Autodesk Inventor part; units mm, degrees
ref_plane "c1_XY" through (22.225, 7.9057, 0) normal (0, 0, 1) x (1, 0, 0)
ref_plane "c1_YZ" through (22.225, 7.9057, 0) normal (1, 0, 0) x (0, 1, 0)
ref_plane "c1_ZX" through (22.225, 7.9057, 0) normal (0, 1, 0) x (0, 0, 1)
sketch "Sketch_18" plane through (0, 0, 0) normal (0, 0, 1) x (1, 0, 0)
  line L0 (22.225, 0) -> (0, 0)
  line L1 (0, 0) -> (0, 12.846)
  line L2 (0, 12.846) -> (0.762, 13.6081)
  line L3 (0.762, 13.6081) -> (4.826, 13.6081)
  line L4 (4.826, 13.6081) -> (5.588, 12.846)
  line L5 (5.588, 12.846) -> (6.35, 12.846)
  line L6 (6.35, 12.846) -> (6.35, 14.1097)
  line L7 (6.35, 14.1097) -> (21.463, 14.1097)
  line L8 (21.463, 14.1097) -> (22.225, 13.3477)
  line L9 (22.225, 13.3477) -> (22.225, 0)
  line L10 (22.225, 0) -> (0, 0)
revolve "Revolution1" add sketch "Sketch_18" angle 360 about axis through (22.225, 0, 0) along (1, 0, 0)
sketch "Sketch_15" plane through (0, 0, 0) normal (0, 0, 1) x (1, 0, 0)
  line L0 (38.1, 0) -> (22.225, 0)
  line L1 (22.225, 0) -> (22.225, 7.9057)
  line L2 (22.225, 7.9057) -> (24.6126, 7.9057)
  line L3 (24.6126, 7.9057) -> (24.6126, 7.7279)
  arc A0 (24.6126, 7.7279) -> (25.5016, 6.839) centre (25.5016, 7.7279) ccw
  line L4 (25.5016, 6.839) -> (26.7843, 6.839)
  arc A1 (26.7843, 6.839) -> (27.383, 7.0708) centre (26.7843, 7.7279) ccw
  line L5 (27.383, 7.0708) -> (27.4129, 7.098)
  line L6 (27.4129, 7.098) -> (28.2524, 7.9375)
  line L7 (28.2524, 7.9375) -> (37.2605, 7.9375)
  line L8 (37.2605, 7.9375) -> (38.1, 7.098)
  line L9 (38.1, 7.098) -> (38.1, 0)
  line L10 (38.1, 0) -> (22.225, 0)
revolve "Revolution2" add sketch "Sketch_15" angle 360 about axis through (38.1, 0, 0) along (1, 0, 0)
thread "Thread1"
sketch "Sketch_9" plane through (38.1, 0, 0) normal (1, 0, 0) x (0, 0, -1)
  line L0 (-28.2194, -56.4388) -> (28.2194, -56.4388)
  line L1 (28.2194, -56.4388) -> (28.2194, 56.4388)
  line L2 (28.2194, 56.4388) -> (-28.2194, 56.4388)
  line L3 (-28.2194, 56.4388) -> (-28.2194, -56.4388)
  line L4 (-4.7307, -28.2194) -> (4.7307, -28.2194)
  line L5 (4.7307, -28.2194) -> (4.7307, 28.2194)
  line L6 (4.7307, 28.2194) -> (-4.7307, 28.2194)
  line L7 (-4.7307, 28.2194) -> (-4.7307, -28.2194)
extrude "Extrusion1" cut sketch "Sketch_9" against normal blind 15.875
sketch "Sketch_13" plane through (0, 0, 0) normal (0, 0, 1) x (1, 0, 0)
  line L0 (21.7996, 0) -> (0, 0)
  line L1 (0, 0) -> (0, 4.7625)
  line L2 (0, 4.7625) -> (19.05, 4.7625)
  line L3 (19.05, 4.7625) -> (21.7996, 0)
  line L4 (21.7996, 0) -> (0, 0)
revolve "Revolution3" cut sketch "Sketch_13" angle 360 about axis through (21.7996, 0, 0) along (1, 0, 0)
sketch "Sketch_19" plane through (0, 0, 0) normal (0, 1, 0) x (-1, 0, 0)
  line L0 (-15.0876, 14.1097) -> (-15.0876, 0)
  line L1 (-15.0876, 0) -> (-19.6754, 0)
  line L2 (-19.6754, 0) -> (-19.6754, 6.0491)
  line L3 (-19.6754, 6.0491) -> (-19.9073, 13.4747)
  line L4 (-19.9073, 13.4747) -> (-20.5423, 14.1097)
  line L5 (-20.5423, 14.1097) -> (-15.0876, 14.1097)
  line L6 (-15.0876, 14.1097) -> (-15.0876, 0)
revolve "Revolution4" cut sketch "Sketch_19" angle 360 about axis through (15.0876, 0, 14.1097) along (0, 0, 1)
sketch "Sketch_24" plane through (0, 0, 0) normal (0, 0, 1) x (1, 0, 0)
  line L0 (6.35, 0) -> (5.588, 0)
  line L1 (5.4861, 14.0255) -> (6.2275, 13.2842)
  arc A0 (6.2275, 13.1046) -> (6.2275, 13.2842) centre (6.1377, 13.1944) ccw
  line L2 (6.2275, 13.1046) -> (5.969, 12.846)
  line L3 (5.969, 12.846) -> (5.588, 12.846)
  line L4 (5.588, 12.846) -> (5.588, 12.5921)
  line L5 (5.588, 12.5921) -> (6.35, 12.5921)
  line L6 (6.35, 12.5921) -> (6.35, 13.449)
  line L7 (6.35, 13.449) -> (5.6893, 14.1097)
  line L8 (5.6893, 14.1097) -> (5.4861, 14.1097)
  line L9 (5.4861, 14.1097) -> (5.4861, 14.0255)
revolve "Revolution5" add sketch "Sketch_24" angle 360 about axis through (6.35, 0, 0) along (1, 0, 0)
sketch "Sketch_43" plane through (0, 0, 0) normal (0, 0, 1) x (1, 0, 0)
  circle A0 centre (30.9626, 0) radius 3.2004
extrude "Extrusion2" cut sketch "Sketch_43" along normal mid plane 14.1922
ref_plane "c1_XY" through (22.225, 7.9057, 0) normal (0, 0, 1) x (1, 0, 0)
ref_plane "c1_YZ" through (22.225, 7.9057, 0) normal (1, 0, 0) x (0, 1, 0)
ref_plane "c1_ZX" through (22.225, 7.9057, 0) normal (0, 1, 0) x (0, 0, 1)
ref_plane "cc1_XY" through (22.225, 0, 0) normal (0, 0, 1) x (1, 0, 0)
ref_plane "cc1_YZ" through (22.225, 0, 0) normal (1, 0, 0) x (0, 1, 0)
ref_plane "cc1_ZX" through (22.225, 0, 0) normal (0, 1, 0) x (0, 0, 1)
ref_plane "c2_XY" through (22.225, -7.9057, 0) normal (0, 0, 1) x (1, 0, 0)
ref_plane "c2_YZ" through (22.225, -7.9057, 0) normal (1, 0, 0) x (0, 1, 0)
ref_plane "c2_ZX" through (22.225, -7.9057, 0) normal (0, 1, 0) x (0, 0, 1)
ref_plane "cc2_XY" through (24.6126, 0, 0) normal (0, 0, 1) x (1, 0, 0)
ref_plane "cc2_YZ" through (24.6126, 0, 0) normal (1, 0, 0) x (0, 1, 0)
ref_plane "cc2_ZX" through (24.6126, 0, 0) normal (0, 1, 0) x (0, 0, 1)
ref_plane "to_tube_XY" through (5.588, 0, 0) normal (1, 0, 0) x (0, 0, -1)
ref_plane "to_tube_YZ" through (5.588, 0, 0) normal (0, 0, -1) x (0, 1, 0)
ref_plane "to_tube_ZX" through (5.588, 0, 0) normal (0, 1, 0) x (1, 0, 0)
ref_plane "to_nut_XY" through (22.225, 0, 0) normal (1, 0, 0) x (0, 0, -1)
ref_plane "to_nut_YZ" through (22.225, 0, 0) normal (0, 0, -1) x (0, 1, 0)
ref_plane "to_nut_ZX" through (22.225, 0, 0) normal (0, 1, 0) x (1, 0, 0)
ref_plane "lovra1_XY" through (33.3248, 0, 0) normal (1, 0, 0) x (0, 0, -1)
ref_plane "lovra1_YZ" through (33.3248, 0, 0) normal (0, 0, -1) x (0, 1, 0)
ref_plane "lovra1_ZX" through (33.3248, 0, 0) normal (0, 1, 0) x (1, 0, 0)
ref_plane "lovra2_XY" through (33.3248, 11.049, 0) normal (1, 0, 0) x (0, 0, -1)
ref_plane "lovra2_YZ" through (33.3248, 11.049, 0) normal (0, 0, -1) x (0, 1, 0)
ref_plane "lovra2_ZX" through (33.3248, 11.049, 0) normal (0, 1, 0) x (1, 0, 0)
ref_plane "lovra3_XY" through (33.3248, -11.049, 0) normal (1, 0, 0) x (0, 0, -1)
ref_plane "lovra3_YZ" through (33.3248, -11.049, 0) normal (0, 0, -1) x (0, 1, 0)
ref_plane "lovra3_ZX" through (33.3248, -11.049, 0) normal (0, 1, 0) x (1, 0, 0)
ref_plane "to_pin_XY" through (30.9626, 0, 0) normal (0, 0, 1) x (1, 0, 0)
ref_plane "to_pin_YZ" through (30.9626, 0, 0) normal (1, 0, 0) x (0, 1, 0)
ref_plane "to_pin_ZX" through (30.9626, 0, 0) normal (0, 1, 0) x (0, 0, 1)
ref_plane "olen_XY" through (30.9626, 0, 0) normal (1, 0, 0) x (0, 0, -1)
ref_plane "olen_YZ" through (30.9626, 0, 0) normal (0, 0, -1) x (0, 1, 0)
ref_plane "olen_ZX" through (30.9626, 0, 0) normal (0, 1, 0) x (1, 0, 0)
ref_plane "thd1_XY" through (38.1, 0, 7.9375) normal (1, 0, 0) x (0, 0, -1)
ref_plane "thd1_YZ" through (38.1, 0, 7.9375) normal (0, 0, -1) x (0, 1, 0)
ref_plane "thd1_ZX" through (38.1, 0, 7.9375) normal (0, 1, 0) x (1, 0, 0)
ref_plane "p1_XY" through (38.1, 0, 4.7307) normal (1, 0, 0) x (0, 0, -1)
ref_plane "p1_YZ" through (38.1, 0, 4.7307) normal (0, 0, -1) x (0, 1, 0)
ref_plane "p1_ZX" through (38.1, 0, 4.7307) normal (0, 1, 0) x (1, 0, 0)
ref_plane "thd2_XY" through (38.1, 0, -7.9375) normal (1, 0, 0) x (0, 0, -1)
ref_plane "thd2_YZ" through (38.1, 0, -7.9375) normal (0, 0, -1) x (0, 1, 0)
ref_plane "thd2_ZX" through (38.1, 0, -7.9375) normal (0, 1, 0) x (1, 0, 0)
ref_plane "p2_XY" through (38.1, 0, -4.7307) normal (1, 0, 0) x (0, 0, -1)
ref_plane "p2_YZ" through (38.1, 0, -4.7307) normal (0, 0, -1) x (0, 1, 0)
ref_plane "p2_ZX" through (38.1, 0, -4.7307) normal (0, 1, 0) x (1, 0, 0)
ref_plane "port2_XY" through (38.1, 0, 0) normal (1, 0, 0) x (0, 0, -1)
ref_plane "port2_YZ" through (38.1, 0, 0) normal (0, 0, -1) x (0, 1, 0)
ref_plane "port2_ZX" through (38.1, 0, 0) normal (0, 1, 0) x (1, 0, 0)
ref_plane "port_XY" through (15.0876, 0, 0) normal (0, 0, 1) x (1, 0, 0)
ref_plane "port_YZ" through (15.0876, 0, 0) normal (1, 0, 0) x (0, 1, 0)
ref_plane "port_ZX" through (15.0876, 0, 0) normal (0, 1, 0) x (0, 0, 1)
ref_plane "1_XY" through (22.225, 0, 0) normal (1, 0, 0) x (0, 0, -1)
ref_plane "1_YZ" through (22.225, 0, 0) normal (0, 0, -1) x (0, 1, 0)
ref_plane "1_ZX" through (22.225, 0, 0) normal (0, 1, 0) x (1, 0, 0)
ref_plane "lovra21_XY" through (0, 0, 5.2705) normal (1, 0, 0) x (0, 0, -1)
ref_plane "lovra21_YZ" through (0, 0, 5.2705) normal (0, 0, -1) x (0, 1, 0)
ref_plane "lovra21_ZX" through (0, 0, 5.2705) normal (0, 1, 0) x (1, 0, 0)
ref_plane "lovra22_XY" through (0, 0, -5.2705) normal (1, 0, 0) x (0, 0, -1)
ref_plane "lovra22_YZ" through (0, 0, -5.2705) normal (0, 0, -1) x (0, 1, 0)
ref_plane "lovra22_ZX" through (0, 0, -5.2705) normal (0, 1, 0) x (1, 0, 0)
ref_plane "to_screw_XY" through (15.0876, 10.2743, -7.0612) normal (0, 1, 0) x (1, 0, 0)
ref_plane "to_screw_YZ" through (15.0876, 10.2743, -7.0612) normal (1, 0, 0) x (0, 0, -1)
ref_plane "to_screw_ZX" through (15.0876, 10.2743, -7.0612) normal (0, 0, -1) x (0, 1, 0)
ref_plane "to_mounting_bracket_XY" through (22.225, 0, 0) normal (1, 0, 0) x (0, 0, -1)
ref_plane "to_mounting_bracket_YZ" through (22.225, 0, 0) normal (0, 0, -1) x (0, 1, 0)
ref_plane "to_mounting_bracket_ZX" through (22.225, 0, 0) normal (0, 1, 0) x (1, 0, 0)
properties part number "09P0010_rear_head"
The model under review builds one solid part; all positions refer to its coordinate system, in mm. A direction names the side the tool comes from. Round coordinates to 2 decimals unless told otherwise and drop trailing zeros. Order: outer loops, then holes, each group sorted by start corner. A loop starts at its lowest first (then second) coordinate and runs counter-clockwise, first axis right, second up. Notation, with made-up numbers: M 8,67.25 L 44,67.25 A28 ccw 44,88.25 Z; hole C -27,11.5 d10. An arc over 180 degrees is marked long. Use a Markdown table: item, result.
1) Insertion check: pin 1 (10 mm diameter, centred on x = 30, z = -6.5, fed in from +Y); pin 2 (6 mm diameter, centred on x = 31, z = -7, fed in from +Y); pin 3 (10 mm diameter, centred on x = 33.5, z = 2, fed in from +Y). Each pin has a flat end and moves straight along its axis. Give the tip position at first contact, or say it passes through.
Report:
| item | result |
|---|---|
| pin 1 | y = 7.79 |
| pin 2 | y = 6.86 |
| pin 3 | y = 7.94 |
2) Consider section C-C (y = -1.5). Give the number of separate pieces and of enclosed holes in the cut face, then the cut area to 3 significant figures.
Report:
| item | result |
|---|---|
| separate pieces | 3 |
| enclosed holes | 0 |
| area | 444 mm^2 |
3) Wall thickness on line 1 along Z through (x, y) = (4.75, 0); line 2 along Z through (x, y) = (11.5, 0); line 3 along Z through (x, y) = (10, -4): over which ranges is each line inside the solid? List them lowest first. Write a range as [from, to].
Report:
| item | result |
|---|---|
| line 1 | [-13.61, -4.76], [4.76, 13.61] |
| line 2 | [-14.11, -4.76] |
| line 3 | [-13.53, -2.58], [2.58, 13.53] |
4) Draft analysis for pull direction Z (two halves, no side actions). For faces 1 (the face through (5.78, -2.78, -12.54)), 2 (the face through (37.954, 7.243, 0.074)), 3 (the face through (11.35, -2.86, 9.81)), state which applies: released by +Z, released by -Z, zero draft, split by the parting line, or undercut.
Report:
| item | result |
|---|---|
| face 1 | undercut |
| face 2 | split by the parting line |
| face 3 | released by +Z |
5) Tool access review of faces 4 (the face through (27.559, 7.243, -0.074)), 5 (the face through (32.82, 7.937, -0.071)), 6 (the face through (20.02, -0.07, 13.59)): name each direction out of +Z, -Z, +X, -X, +Y, -Y from which nothing blocks a thin tool from reaching the whole face with its end or side.
Report:
| item | result |
|---|---|
| face 4 | +Y |
| face 5 | +X, +Y |
| face 6 | +Z |
6) Consider section B-B (x = 8.5). Write out the cut boundary in (y, z) (1 decimal), then the cut area to 3 significant figures.
Report:
| item | result |
|---|---|
| outline | C 0,0 d28.2; hole C 0,0 d9.5 |
| area | 554 mm^2 |
7) Consider section A-A (x = 30.5). Write out the cut boundary in (y, z) (1 decimal).
Report:
| item | result |
|---|---|
| outline | M -6.4,-4.7 L -3.2,-4.7 L -3.2,4.7 L -6.4,4.7 A7.9 ccw Z; M 3.2,-4.7 L 6.4,-4.7 A7.9 ccw 6.4,4.7 L 3.2,4.7 Z |
